from build123d import *

# Parameters (mm, degrees)
SKETCH_R        = 15
PAD_DEPTH       = 25
SKETCH001_R     = 12.75
POCKET_DEPTH    = 20
CHAMFER_SIZE    = 2
CHAMFER001_SIZE = 1


with BuildPart() as part:
    # Sketch (on XY_Plane of Origin) → Pad (new body)
    with BuildSketch(Plane.XY):
        Circle(SKETCH_R)
    extrude(amount=PAD_DEPTH)

    # Sketch001 (on Face3 of Pad) → Pocket (cut)
    with BuildSketch(Plane.XY.offset(25)):
        Circle(SKETCH001_R)
    extrude(amount=-POCKET_DEPTH, mode=Mode.SUBTRACT)

    # Chamfer
    chamfer_edges = [part.edges().sort_by_distance(p)[0] for p in [
        (-15, 0, 0),
    ]]
    chamfer(chamfer_edges, length=CHAMFER_SIZE)

    # Chamfer001
    chamfer001_edges = [part.edges().sort_by_distance(p)[0] for p in [
        (-12.75, 0, 25),
    ]]
    chamfer(chamfer001_edges, length=CHAMFER001_SIZE)


solid = part.part
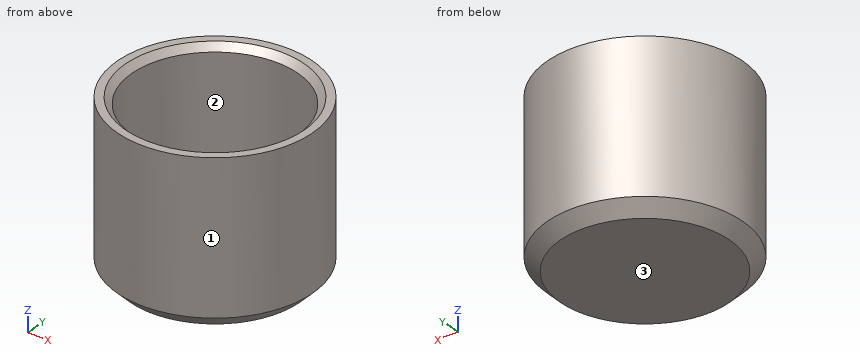
Check sheet for the modelled part. Datum: model origin and axes. Units: mm. Face numbers are marked on the shaded views. Round coordinates to 2 decimals unless told otherwise and drop trailing zeros. Loops run counter-clockwise (first coordinate to the right, second up) from the corner with the lowest first, then second, coordinate; pieces in that order, holes last. Notation, with made-up numbers: (3, 87) - (25, 87) arc R9 cw to (25, 103) - close; hole circle Ø7 at (39.25, -21.75). An arc over 180 degrees is marked (long way). Answer as CSV lines item,"result". Start each with the question number.
Item 1: Section check C-C (z = 7). Record the boundary of the cut face in (x, y), and give its area (3 significant figures).
Item 2: Depth check by flat-ended pin: P1, Ø5, axis at x = 1, y = 9, coming from the +Z side; P2, Ø1, axis at x = 9.5, y = 11.5, coming from the -Z side; P3, Ø4, axis at x = -5.5, z = 4, coming from the -Y side. Enter the tip coordinate at first touch or a pass-through.
Item 3: Section check A-A (x = 0). Record the boundary of the cut face in (y, z).
Item 4: Section check D-D (z = 3.75). Record the boundary of the cut face in (x, y), and give its area (3 significant figures).
Item 5: Release check for a two-part mould opening along X. For the marked faces 1, 2 and 3 record: +X half, -X half, draft (parallel to the pull), parting line (faces both ways), or undercut.
Item 6: Scan lines: line 1 (Y direction, x = 0, z = 9); line 2 (Z direction, x = 10, y = 7.5); line 3 (X direction, y = -1, z = 18.5). Record each from-to range of solid material in increasing order. Write a range as [from, to].
Report:
1,outline,"circle Ø30 at (0, 0); hole circle Ø25.5 at (0, 0)"
1,area,"196 mm2"
2,P1,"stops at z = 5"
2,P2,"stops at z = 1.42"
2,P3,"stops at y = -14.59"
3,outline,"(-15, 2) - (-13, 0) - (13, 0) - (15, 2) - (15, 25) - (13.75, 25) - (12.75, 24) - (12.75, 5) - (-12.75, 5) - (-12.75, 24) - (-13.75, 25) - (-15, 25) - close"
4,outline,"circle Ø30 at (0, 0)"
4,area,"707 mm2"
5,face 1,"parting line"
5,face 2,"undercut"
5,face 3,"draft"
6,line 1,"y = [-15, -12.75], [12.75, 15]"
6,line 2,"z = [0, 5]"
6,line 3,"x = [-14.97, -12.71], [12.71, 14.97]"
